The listing builds one solid part. Answer for the finished solid, in the listing's coordinates (mm). A direction names the side the tool comes from. Round coordinates to 2 decimals unless told otherwise and drop trailing zeros. Write each loop counter-clockwise with the first axis right and the second up, starting at its lowest first coordinate (ties: lowest second). Pieces come first, ordered by that corner, then holes. Notation, with made-up numbers: (85.25, -31) - (104.25, -31) arc R27 ccw to (104.25, 8) - close; hole circle Ø3 at (24.25, 72). An arc over 180 degrees is marked (long way). Answer as CSV lines item,"result". Start each with the question number.
Item 1: A cutting plane is placed at C-C on x = 130. Determine the outline of the cut face in (y, z).
Item 2: Straight lines are drawn through the part: line 1 along Z through (x, y) = (158.75, 14); line 2 along X through (y, z) = (5.5, -152.4); line 3 along X through (y, z) = (29.5, -165). For each, find the intervals that lie inside material, in ascending order. Write a range as [from, to].
Item 3: A cutting plane is placed at A-A on y = 31. Determine the outline of the cut face in (x, z), and give its area (3 significant figures).
Item 4: Flat-ended cylindrical pins translate along their axes: pin 1 (4.5 mm diameter, centred on x = 158.75, z = -101.6, fed in from +Y); pin 2 (8 mm diameter, centred on x = 95.25, z = -152.4, fed in from +Y). Find the tip coordinate at first contact, or state that the pin passes through.
Item 5: Which of the six approach directions +Z, -Z, +X, -X, +Y, -Y give full straight-line access (tool end or side, diameter ignored) to faces 1 (the flat face through (254, 19, -125)), 2 (the flat face through (126, 32, -76.2))?
Item 6: For a pull along Z with two mould halves and no side action, classify faces 3 (the flat face through (125, 19, -254)), 4 (the flat face through (125, 38.1, -72)), 5 (the flat face through (128, 32, -177.8)), 6 (the cylindrical face through (65.31, 31.84, -78.11)) as pulls with the +Z half, pulls with the -Z half, needs draft (parallel to the pull), parting line crosses it, or undercut.
Item 7: A cutting plane is placed at B-B on z = -126.5. Determine the outline of the cut face in (x, y), and give its area (3 significant figures).
```python
from build123d import *

# Parameters (mm, degrees)
SKETCH1_W               = 254
SKETCH1_H               = 254
BOSS_EXTRUDE1_DEPTH     = 38.1
CUT_EXTRUDE1_DEPTH      = 12.7
CUT_EXTRUDE2_DEPTH      = 361.10715072
CUT_EXTRUDE2_DEPTH_BACK = 361.10715072
SKETCH4_R               = 2.4638
CHAMFER1_SIZE           = 12.7


with BuildPart() as part:
    # Sketch1 → Boss-Extrude1 (new body)
    with BuildSketch(Plane(origin=(0, 0, 0), x_dir=(1, 0, 0), z_dir=(0, 1, 0))):
        with Locations((127, 127)):
            Rectangle(SKETCH1_W, SKETCH1_H)
    extrude(amount=BOSS_EXTRUDE1_DEPTH)

    # Sketch2 → Cut-Extrude1 (cut)
    with BuildSketch(Plane(origin=(0, 38.1, 0), x_dir=(1, 0, 0), z_dir=(0, 1, 0))):
        with BuildLine():
            Line((69.85, 76.2), (184.15, 76.2))
            ThreePointArc((184.15, 76.2), (188.640128061, 78.059871939), (190.5, 82.55))
            Line((190.5, 82.55), (190.5, 171.45))
            ThreePointArc((190.5, 171.45), (188.640128061, 175.940128061), (184.15, 177.8))
            Line((184.15, 177.8), (69.85, 177.8))
            ThreePointArc((69.85, 177.8), (65.359871939, 175.940128061), (63.5, 171.45))
            Line((63.5, 171.45), (63.5, 82.55))
            ThreePointArc((63.5, 82.55), (65.359871939, 78.059871939), (69.85, 76.2))
        make_face()
    extrude(amount=-CUT_EXTRUDE1_DEPTH, mode=Mode.SUBTRACT)

    # Sketch4 → Cut-Extrude2 (cut, two sides: drawn at the far end of the back side and taken through both)
    with BuildSketch(Plane(origin=(0, 25.4, 0), x_dir=(1, 0, 0), z_dir=(0, 1, 0)).offset(-CUT_EXTRUDE2_DEPTH_BACK)):
        with Locations(Location((95.25, 152.4, 0), (0, 0, 270))):
            Circle(SKETCH4_R)
        with Locations(Location((158.75, 152.4, 0), (0, 0, 270))):
            Circle(SKETCH4_R)
        with Locations(Location((158.75, 101.6, 0), (0, 0, 270))):
            Circle(SKETCH4_R)
        with Locations(Location((95.25, 101.6, 0), (0, 0, 270))):
            Circle(SKETCH4_R)
    extrude(amount=CUT_EXTRUDE2_DEPTH + CUT_EXTRUDE2_DEPTH_BACK, mode=Mode.SUBTRACT)

    # Chamfer1
    chamfer1_edges = [part.edges().sort_by_distance(p)[0] for p in [
        (0, 19.05, -254),
        (0, 19.05, 0),
        (254, 19.05, 0),
        (254, 19.05, -254),
    ]]
    chamfer(chamfer1_edges, length=CHAMFER1_SIZE)


solid = part.part
```
Geometry says:
1,outline,"(0, -254) - (38.1, -254) - (38.1, -177.8) - (25.4, -177.8) - (25.4, -76.2) - (38.1, -76.2) - (38.1, 0) - (0, 0) - close"
2,line 1,"z = [-254, -154.86], [-149.94, -104.06], [-99.14, 0]"
2,line 2,"x = [0, 92.79], [97.71, 156.29], [161.21, 254]"
2,line 3,"x = [0, 63.5], [190.5, 254]"
3,outline,"(0, -241.3) - (12.7, -254) - (241.3, -254) - (254, -241.3) - (254, -12.7) - (241.3, 0) - (12.7, 0) - (0, -12.7) - close; hole (63.5, -171.45) arc R6.35 ccw to (69.85, -177.8) - (184.15, -177.8) arc R6.35 ccw to (190.5, -171.45) - (190.5, -82.55) arc R6.35 ccw to (184.15, -76.2) - (69.85, -76.2) arc R6.35 ccw to (63.5, -82.55) - close"
3,area,"51,300 mm^2"
4,pin 1,"passes through"
4,pin 2,"stops at y = 25.4"
5,face 1,"+Z, -Z, +X, +Y, -Y"
5,face 2,"+Y"
6,face 3,"pulls with the -Z half"
6,face 4,"needs draft"
6,face 5,"undercut"
6,face 6,"undercut"
7,outline,"(0, 0) - (254, 0) - (254, 38.1) - (190.5, 38.1) - (190.5, 25.4) - (63.5, 25.4) - (63.5, 38.1) - (0, 38.1) - close"
7,area,"8,060 mm^2"
